```python
from build123d import *

# Parameters (mm, degrees)
AUFSATZ_LINEAR_AUSTRAGEN1_DEPTH                      = 4
VERRUNDUNG1_R                                        = 5
FORMSENKUNG_F_R_M3_SENKSCHRAUBE_MIT_INNE_D           = 2
FORMSENKUNG_F_R_M3_SENKSCHRAUBE_MIT_INNE_CSINK_D     = 3.5
FORMSENKUNG_F_R_M3_SENKSCHRAUBE_MIT_INNE_CSINK_ANGLE = 90
M2_GEWINDEBOHRUNG1_D                                 = 1.6


with BuildPart() as part:
    # Skizze1 → Aufsatz-Linear austragen1 (new body)
    with BuildSketch(Plane(origin=(0, 0, 0), x_dir=(1, 0, 0), z_dir=(0, 1, 0))):
        Polygon((-15, 15), (-15, -15), (15, -15), (15, 15), (15, 24), (-15, 24), align=None)
        Polygon((-12.5, 7.5), (-7.5, 7.5), (-7.5, 12.5), (7.5, 12.5), (7.5, 7.5), (12.5, 7.5), (12.5, -7.5), (7.5, -7.5), (7.5, -12.5), (-7.5, -12.5), (-7.5, -7.5), (-12.5, -7.5), align=None, mode=Mode.SUBTRACT)
    extrude(amount=AUFSATZ_LINEAR_AUSTRAGEN1_DEPTH)

    # Verrundung1
    verrundung1_edges = [part.edges().sort_by_distance(p)[0] for p in [
        (-7.5, 2, 12.5),
        (-12.5, 2, 7.5),
        (12.5, 2, 7.5),
        (7.5, 2, 12.5),
        (12.5, 2, -7.5),
        (7.5, 2, -12.5),
        (-7.5, 2, -12.5),
        (-12.5, 2, -7.5),
    ]]
    fillet(verrundung1_edges, radius=VERRUNDUNG1_R - 0.0001)  # a hair under: the kernel refuses the full size

    # Formsenkung für M3 Senkschraube mit Innensechskant1 (through all)
    with Locations(Plane(origin=(0, 4, 0), x_dir=(1, 0, 0), z_dir=(0, 1, 0))):
        with Locations((-10, 20), (10, 20)):
            CounterSinkHole(FORMSENKUNG_F_R_M3_SENKSCHRAUBE_MIT_INNE_D / 2, FORMSENKUNG_F_R_M3_SENKSCHRAUBE_MIT_INNE_CSINK_D / 2, counter_sink_angle=FORMSENKUNG_F_R_M3_SENKSCHRAUBE_MIT_INNE_CSINK_ANGLE)

    # M2 Gewindebohrung1 (through all)
    with Locations(Plane(origin=(0, 4, 0), x_dir=(1, 0, 0), z_dir=(0, 1, 0))):
        with Locations((-10, 10), (10, 10), (10, -10), (-10, -10)):
            Hole(M2_GEWINDEBOHRUNG1_D / 2)


solid = part.part
```
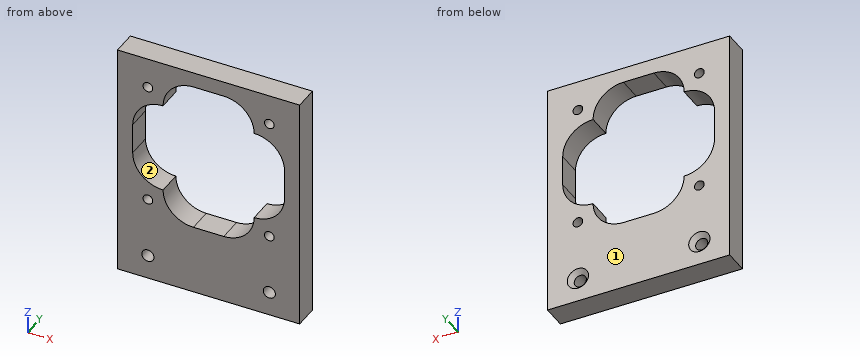
Input: part model. Units: mm. Frame: model coordinates. Face numbers are marked on the shaded views. A direction names the side the tool comes from. Round coordinates to 2 decimals unless told otherwise and drop trailing zeros. Order: outer loops, then holes, each group sorted by start corner. A loop starts at its lowest first (then second) coordinate and runs counter-clockwise, first axis right, second up. Notation, with made-up numbers: (84.25, -40) - (119.25, -40) arc R36 ccw to (119.25, -2) - close; hole circle Ø3 at (-7.75, 4.25). An arc over 180 degrees is marked (long way). One line per question, with ' | ' between items. Start each with the question number.
1) Contact query for a flat-ended pin moving along its axis: P1, Ø3, axis at x = -10, z = -20, coming from the -Y side. Output: stop coordinate, or through.
2) Ray query, probe 1 along Z at (x, y) = (10, 0.7); probe 2 along X at (y, z) = (3, -10); probe 3 along Z at (x, y) = (2.25, 0.95). Return the intervals inside material, ascending.
3) Cut plane D-D, the plane x = -10. Return the cut outline in (y, z), then the cut area to 3 significant figures.
4) Cut plane C-C, the plane z = 5. Return the cut outline in (x, y), then the cut area to 3 significant figures.
5) Cut plane B-B, the plane y = 1.5. Give the number of separate pieces and of enclosed holes in the cut face, then the cut area to 3 significant figures.
6) Cut plane A-A, the plane x = 0.75. Return the cut outline in (y, z), then the cut area to 3 significant figures.
7) Set-up query: the marked faces 1 and 2. Return all of +Z, -Z, +X, -X, +Y, -Y with unobstructed straight access to the full face (end or side cutting, diameter ignored); none if empty.
Worked out:
1) P1: stops at y = 0
2) probe 1: z = -24 to -21, -19 to -10.8, -9.2 to -6.83, 6.83 to 9.2, 10.8 to 15 | probe 2: x = -15 to -10.8, -9.2 to -6.83, 6.83 to 9.2, 10.8 to 15 | probe 3: z = -24 to -12.5, 12.5 to 15
3) outline: (0, -24) - (4, -24) - (4, -21.75) - (3.25, -21) - (0, -21) - close; (0, -19) - (3.25, -19) - (4, -18.25) - (4, -10.8) - (0, -10.8) - close; (0, -9.2) - (4, -9.2) - (4, -6.83) - (0, -6.83) - close; (0, 6.83) - (4, 6.83) - (4, 9.2) - (0, 9.2) - close; (0, 10.8) - (4, 10.8) - (4, 15) - (0, 15) - close | area: 80.0 mm^2
4) outline: (-15, 0) - (-11.83, 0) - (-11.83, 4) - (-15, 4) - close; (11.83, 0) - (15, 0) - (15, 4) - (11.83, 4) - close | area: 25.4 mm^2
5) separate pieces: 1 | enclosed holes: 7 | area: 674 mm^2
6) outline: (0, -24) - (4, -24) - (4, -12.5) - (0, -12.5) - close; (0, 12.5) - (4, 12.5) - (4, 15) - (0, 15) - close | area: 56.0 mm^2
7) face 1: +Z, -Z, +X, -X, +Y | face 2: +Y, -Y
